```python
from build123d import *

# Parameters (mm, degrees)
SKETCH1_R           = 1.5
BASEBODY_DEPTH      = 10
BASETOP_FACE_RADIUS = 2.723673019
BASETOP_HEIGHT      = 0.28
SKETCH5_W           = 4
SKETCH5_H           = 2
CROSSRECESS_DEPTH   = 1.4
FILLET1_R           = 0.2
DRAFT3_ANGLE        = -10


# Read off the part's stored shape, not the designer's step: Neck, BaseHead
with BuildPart() as part:
    # Sketch1 → BaseBody (new body)
    with BuildSketch(Plane(origin=(0, 0, 0), x_dir=(0, 0, -1), z_dir=(1, 0, 0))):
        Circle(SKETCH1_R)
    extrude(amount=BASEBODY_DEPTH)

    # Neck outline → Neck (revolve, cut)
    with BuildSketch(Plane.YX):
        Polygon((1.5, 2.4), (1.076815246, 0), (1.5, 0), align=None)
    revolve(axis=Axis((0, 0, 0), (1, 0, 0)), mode=Mode.SUBTRACT)

    # BaseHead outline → BaseHead (revolve)
    with BuildSketch(Plane.YX):
        Polygon((0, 0), (2.723673019, 0), (1.323673019, 1.4), (0, 1.4), align=None)
    revolve(axis=Axis((0, 0, 0), (1, 0, 0)))

    # BaseTop: a dome of height H over a round flat face of radius A is a cap of a sphere of radius (A * A + H * H) / (2 * H)
    basetop_r = (BASETOP_FACE_RADIUS * BASETOP_FACE_RADIUS + BASETOP_HEIGHT * BASETOP_HEIGHT) / (2 * BASETOP_HEIGHT)
    basetop_base = Plane((0, 0, 0), z_dir=(-1, 0, 0))
    with Locations(basetop_base.offset(BASETOP_HEIGHT - basetop_r)):
        basetop_ball = Sphere(basetop_r, mode=Mode.PRIVATE)
    add(split(basetop_ball, bisect_by=basetop_base, keep=Keep.TOP, mode=Mode.PRIVATE))

    # Sketch5 → Cut-Revolve1 (revolve, cut)
    with BuildSketch(Plane.XY):
        with Locations((0, 3.68)):
            Rectangle(SKETCH5_W, SKETCH5_H)
    revolve(axis=Axis((10, 0, 0), (-1, 0, 0)), mode=Mode.SUBTRACT)

    # Sketch7 → CrossRecess (cut)
    with BuildSketch(Plane(origin=(-0.28, 0, 0), x_dir=(0, 0, -1), z_dir=(1, 0, 0))):
        Polygon((0.27, -0.27), (0.27, -1.35), (-0.27, -1.35), (-0.27, -0.27), (-1.35, -0.27), (-1.35, 0.27), (-0.27, 0.27), (-0.27, 1.35), (0.27, 1.35), (0.27, 0.27), (1.35, 0.27), (1.35, -0.27), align=None)
    extrude(amount=CROSSRECESS_DEPTH, mode=Mode.SUBTRACT)

    # Fillet1
    fillet1_edges = [part.edges().sort_by_distance(p)[0] for p in [
        (0.422723318, 0.27, 0.27),
        (0.422723318, -0.27, 0.27),
        (0.422723318, -0.27, -0.27),
        (0.422723318, 0.27, -0.27),
    ]]
    fillet(fillet1_edges, radius=FILLET1_R)

    # Draft3
    draft3_faces = [part.faces().sort_by_distance(p)[0] for p in [
        (0.454577412, -1.35, 0),
        (0.454577412, 0, 1.35),
        (0.454577412, 0, -1.35),
        (0.454577412, 1.35, 0),
    ]]
    draft(draft3_faces, Plane(origin=(-0.28, 0, 0), x_dir=(0, 0, 1), z_dir=(1, 0, 0)), DRAFT3_ANGLE)

    # Sketch8 → Cut-Revolve2 (revolve, cut)
    with BuildSketch(Plane.XY, mode=Mode.PRIVATE) as cut_revolve2_sk:
        with BuildLine():
            Line((1.4, 1.323673019), (0.043673019, 2.68))
            Line((0.043673019, 2.68), (2.4, 2.68))
            Line((2.4, 2.68), (2.4, 1.5))
            Line((2.4, 1.5), (1.595834298, 1.272638584))
            ThreePointArc((1.595834298, 1.272638584), (1.490985809, 1.271558189), (1.4, 1.323673019))
        make_face()
    revolve(cut_revolve2_sk.sketch.rotate(Axis((0, 0, 0), (1, 0, 0)), 90), axis=Axis((0, 0, 0), (1, 0, 0)), mode=Mode.SUBTRACT)


solid = part.part
```
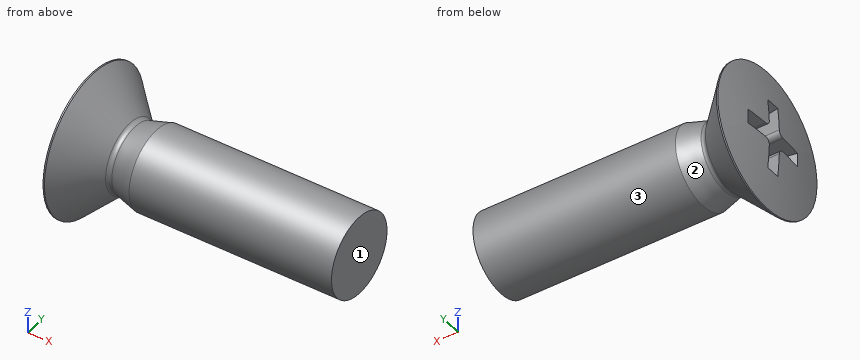
The model under review builds one solid part; all positions refer to its coordinate system, in mm. Face numbers are marked on the shaded views. Coordinates: 2 decimals unless noted, no trailing zeros. Write each loop counter-clockwise with the first axis right and the second up, starting at its lowest first coordinate (ties: lowest second). Pieces come first, ordered by that corner, then holes. Notation, with made-up numbers: (-35, 17.25) - (21, 17.25) arc R15 cw to (21, 31.25) - close; hole circle Ø6 at (27.25, 0). An arc over 180 degrees is marked (long way). Answer in a Markdown table with one row per item. Add a question column.
Q1. Draft analysis for pull direction X (two halves, no side actions). For the marked faces 1, 2 and 3, state which applies: +X half, -X half, draft (parallel to the pull), parting line (faces both ways), or undercut.
Q2. To check wall thickness, follow line 1 along X through (y, z) = (0.9, 1.25); line 2 along X through (y, z) = (0.45, 0.85); line 3 along Y through (x, z) = (0.75, 1.7). State the ranges of each line that lie inside material, in increasing order. Write a range as from..to.
Q3. Clearance check with flat-ended pins moving along their axes: pin 1 (0.7 mm diameter, centred on x = 0.5, z = -0.5, fed in from -Y); pin 2 (1 mm diameter, centred on x = 0, z = 1, fed in from -Y); pin 3 (2 mm diameter, centred on x = 4.5, y = -0.5, fed in from -Z); pin 4 (1.8 mm diameter, centred on y = -0.5, z = -0.5, fed in from -X). State where each tip first meets the part, or that it passes through.
Q4. Consider section D-D on x = 1.75. Give the boundary of the cut face in (y, z).
Q5. Consider section C-C on x = 3. Give the boundary of the cut face in (y, z), then the cut area to 3 significant figures.
Q6. Consider section A-A on y = 0. Give the boundary of the cut face in (x, z), then the cut area to 3 significant figures.
Answers below:
| question | item | result |
|---|---|---|
| 1 | face 1 | +X half |
| 1 | face 2 | undercut |
| 1 | face 3 | draft |
| 2 | line 1 | -0.19..1.18 |
| 2 | line 2 | -0.25..10 |
| 2 | line 3 | -1..1 |
| 3 | pin 1 | y = -2.53 |
| 3 | pin 2 | y = -2.63 |
| 3 | pin 3 | z = -1.5 |
| 3 | pin 4 | x = -0.27 |
| 4 | outline | circle Ø2.63 at (0, 0) |
| 5 | outline | circle Ø3 at (0, 0) |
| 5 | area | 7.07 mm² |
| 6 | outline | (-0.21, -1.34) arc R13.39 ccw to (-0.01, -2.68) - (0.04, -2.68) - (1.4, -1.32) arc R0.2 cw to (1.6, -1.27) - (2.4, -1.5) - (10, -1.5) - (10, 1.5) - (2.4, 1.5) - (1.6, 1.27) arc R0.2 cw to (1.4, 1.32) - (0.04, 2.68) - (-0.01, 2.68) arc R13.39 ccw to (-0.21, 1.34) - (1.12, 1.1) - (1.12, -1.1) - close |
| 6 | area | 28.8 mm² |
